Geometry check sheet. Reference: the model listing, model coordinates, mm. A direction names the side the tool comes from. Give positions to 0.01 mm unless a question says otherwise; leave off trailing zeros. Order: outer loops, then holes, each group sorted by start corner. A loop starts at its lowest first (then second) coordinate and runs counter-clockwise, first axis right, second up.
```python
from build123d import *

# Parameters (mm, degrees)
AUFSATZ_LINEAR_AUSTRAGEN1_DEPTH = 505
SKIZZE2_R                       = 3.25
SCHNITT_LINEAR_AUSTRAGEN1_DEPTH = 60
SKIZZE3_R                       = 2.75
SCHNITT_LINEAR_AUSTRAGEN2_DEPTH = 100
SKIZZE4_R                       = 15
SCHNITT_LINEAR_AUSTRAGEN3_DEPTH = 100
SKIZZE5_R                       = 2.5
SCHNITT_LINEAR_AUSTRAGEN4_DEPTH = 100
SKIZZE6_R                       = 3
SCHNITT_LINEAR_AUSTRAGEN5_DEPTH = 10
SKIZZE7_R                       = 20
SCHNITT_LINEAR_AUSTRAGEN6_DEPTH = 5


with BuildPart() as part:
    # Skizze1 → Aufsatz-Linear austragen1 (new body)
    with BuildSketch(Plane.XY):
        with BuildLine():
            Line((-34, 20), (34, 20))
            ThreePointArc((34, 20), (38.242640687, 18.242640687), (40, 14))
            Line((40, 14), (40, -14))
            ThreePointArc((40, -14), (38.242640687, -18.242640687), (34, -20))
            Line((34, -20), (-34, -20))
            ThreePointArc((-34, -20), (-38.242640687, -18.242640687), (-40, -14))
            Line((-40, -14), (-40, 14))
            ThreePointArc((-40, 14), (-38.242640687, 18.242640687), (-34, 20))
        make_face()
        with BuildLine():
            Line((-37, 14), (-37, -14))
            ThreePointArc((-37, -14), (-36.121320344, -16.121320344), (-34, -17))
            Line((-34, -17), (34, -17))
            ThreePointArc((34, -17), (36.121320344, -16.121320344), (37, -14))
            Line((37, -14), (37, 14))
            ThreePointArc((37, 14), (36.121320344, 16.121320344), (34, 17))
            Line((34, 17), (-34, 17))
            ThreePointArc((-34, 17), (-36.121320344, 16.121320344), (-37, 14))
        make_face(mode=Mode.SUBTRACT)
    extrude(amount=AUFSATZ_LINEAR_AUSTRAGEN1_DEPTH)

    # Skizze2 → Schnitt-Linear austragen1 (cut)
    with BuildSketch(Plane(origin=(0, 20, 0), x_dir=(1, 0, 0), z_dir=(0, 1, 0))):
        with Locations(Location((20, -369.5, 0), (0, 0, 270))):
            Circle(SKIZZE2_R)
        with Locations(Location((20, -422.5, 0), (0, 0, 270))):
            Circle(SKIZZE2_R)
        with Locations(Location((-20, -422.5, 0), (0, 0, 90))):
            Circle(SKIZZE2_R)
        with Locations(Location((-20, -369.5, 0), (0, 0, 90))):
            Circle(SKIZZE2_R)
    extrude(amount=-SCHNITT_LINEAR_AUSTRAGEN1_DEPTH, mode=Mode.SUBTRACT)

    # Skizze3 → Schnitt-Linear austragen2 (cut)
    with BuildSketch(Plane(origin=(40, 0, 0), x_dir=(0, 0, -1), z_dir=(1, 0, 0))):
        with Locations((-18.5, 0)):
            Circle(SKIZZE3_R)
        with Locations((-59, 0)):
            Circle(SKIZZE3_R)
        with Locations((-99, 0)):
            Circle(SKIZZE3_R)
        with Locations((-131.5, 0)):
            Circle(SKIZZE3_R)
        with Locations((-147.5, 0)):
            Circle(SKIZZE3_R)
    extrude(amount=-SCHNITT_LINEAR_AUSTRAGEN2_DEPTH, mode=Mode.SUBTRACT)

    # Skizze4 → Schnitt-Linear austragen3 (cut)
    with BuildSketch(Plane.XZ.offset(20)):
        with Locations(Location((-12.7, 74.5, 0), (0, 0, 270))):
            Circle(SKIZZE4_R)
    extrude(amount=-SCHNITT_LINEAR_AUSTRAGEN3_DEPTH, mode=Mode.SUBTRACT)

    # Skizze5 → Schnitt-Linear austragen4 (cut)
    with BuildSketch(Plane.ZY.offset(40)):
        with Locations((465, 0)):
            Circle(SKIZZE5_R)
        with Locations((385, 0)):
            Circle(SKIZZE5_R)
        with Locations((305, 0)):
            Circle(SKIZZE5_R)
        with Locations((225, 0)):
            Circle(SKIZZE5_R)
    extrude(amount=-SCHNITT_LINEAR_AUSTRAGEN4_DEPTH, mode=Mode.SUBTRACT)

    # Skizze6 → Schnitt-Linear austragen5 (cut)
    with BuildSketch(Plane.XZ.offset(20)):
        with Locations(Location((-12.7, 41.195270606, 0), (0, 0, 270))):
            Circle(SKIZZE6_R)
        with Locations(Location((20.604729394, 74.5, 0), (0, 0, 270))):
            Circle(SKIZZE6_R)
        with Locations(Location((-12.7, 107.804729394, 0), (0, 0, 270))):
            Circle(SKIZZE6_R)
        with Locations((-46.004729394, 74.5)):
            Circle(SKIZZE6_R)
    extrude(amount=-SCHNITT_LINEAR_AUSTRAGEN5_DEPTH, mode=Mode.SUBTRACT)

    # Skizze7 → Schnitt-Linear austragen6 (cut)
    with BuildSketch(Plane.XZ.offset(20)):
        with Locations(Location((-12.7, 74.5, 0), (0, 0, 270))):
            Circle(SKIZZE7_R)
    extrude(amount=-SCHNITT_LINEAR_AUSTRAGEN6_DEPTH, mode=Mode.SUBTRACT)


solid = part.part
```
Q1. Release check for a two-part mould opening along Y. For faces 1 (the face through (0, -17, 249)), 2 (the face through (0, 20, 249)), 3 (the face through (40, 0, 249)), 4 (the face through (0, -20, 249)) record: pulls with the +Y half, pulls with the -Y half, needs draft (parallel to the pull), parting line crosses it, or undercut.
Q2. Thickness scan on L1, parallel to Y at x = 39.2, z = 305; L2, parallel to Y at x = -6.5, z = 285.5; L3, parallel to X at y = 19.3, z = 369.5. Record the ranges inside material, lowest first.
Q3. Cross-section at B-B, the plane y = -9.5. Record the boundary of the cut face in (x, z), and give its area (3 significant figures).
Q4. Cross-section at A-A, the plane z = 441. Record the boundary of the cut face in (x, y).
Q5. Gauge pin test, flat end, axial feed: P1, Ø7, axis at y = 0, z = 99, coming from the +X side. Record the tip position at first contact, or that the pin passes through.
Q6. Access from +Z, -Z, +X, -X, +Y, -Y to the whole of each face (thin tool, end or side, straight path). Record for faces 5 (the face through (-40, 0, 249)), 6 (the face through (-11.82, -18.52, 94.48)), 7 (the face through (37, 0, 249)).
Answers follow:
1. face 1: undercut
1. face 2: pulls with the +Y half
1. face 3: needs draft
1. face 4: pulls with the -Y half
2. L1: y = -16.99 to -2.5, 2.5 to 16.99
2. L2: y = -20 to -17, 17 to 20
2. L3: x = -36.81 to -23.25, -16.75 to 16.75, 23.25 to 36.81
3. outline: (-40, 0) - (-37, 0) - (-37, 505) - (-40, 505) - close; (37, 0) - (40, 0) - (40, 505) - (37, 505) - close
3. area: 3,030 mm2
4. outline: (-40, -14) arc R6 ccw to (-34, -20) - (34, -20) arc R6 ccw to (40, -14) - (40, 14) arc R6 ccw to (34, 20) - (-34, 20) arc R6 ccw to (-40, 14) - close; hole (-37, -14) arc R3 ccw to (-34, -17) - (34, -17) arc R3 ccw to (37, -14) - (37, 14) arc R3 ccw to (34, 17) - (-34, 17) arc R3 ccw to (-37, 14) - close
5. P1: stops at x = 40
6. face 5: +Z, -Z, -X, +Y, -Y
6. face 6: -Y
6. face 7: +Z, -Z
